Could you check a few things on this model? Use its own coordinates, in mm. A direction names the side the tool comes from. Coordinates: 2 decimals unless noted, no trailing zeros. Order: outer loops, then holes, each group sorted by start corner. A loop starts at its lowest first (then second) coordinate and runs counter-clockwise, first axis right, second up. Notation, with made-up numbers: M 52.25,-22 L 104.25,-22 A22 cw 104.25,9 Z; hole C -22,38 d4. An arc over 180 degrees is marked long. Write item = value, one per line. Start each with the question number.
from build123d import *

# Parameters (mm, degrees)
BOSS_EXTRUDE1_DEPTH = 29.5
SKETCH2_W           = 2
SKETCH2_H           = 1.8
BOSS_EXTRUDE2_DEPTH = 29.5


with BuildPart() as part:
    # Sketch1 → Boss-Extrude1 (new body)
    with BuildSketch(Plane.XY):
        Polygon((-7.65, 2.6), (2.05, 2.6), (2.05, -7), (-1.15, -7), (-1.15, -5), (0.05, -5), (0.05, 0.2), (-5.65, 0.2), (-5.65, -5), (-4.45, -5), (-4.45, -7), (-7.65, -7), align=None)
    extrude(amount=BOSS_EXTRUDE1_DEPTH)

    # Sketch2 → Boss-Extrude2 (add)
    with BuildSketch(Plane.XY.offset(29.5)):
        with Locations((1.05, 3.5)):
            Rectangle(SKETCH2_W, SKETCH2_H)
    extrude(amount=-BOSS_EXTRUDE2_DEPTH)


solid = part.part
(1) Thinking about a two-plate mould opening in Y: for faces 5 (the flat face through (-4, 2.6, 15)), 6 (the flat face through (2.05, -1, 15)), 7 (the flat face through (-0.6, -5, 14.5)), which applies, released by +Y, released by -Y, zero draft, split by the parting line, or undercut?
(2) Imagine slicing it at C-C on z = 10. List the corners of the cut face in (x, y) for me.
(3) For faces 1 (the flat face through (0.05, 3, 15)), 2 (the flat face through (-5.65, -2, 15)), 3 (the flat face through (-1.15, -6, 15)), 4 (the flat face through (-3, 1, 0)), which set-ups out of +Z, -Z, +X, -X, +Y, -Y let a thin tool reach every point of the face, with its end or its side?
(4) Imagine slicing it at D-D on x = -6.75. List the corners of the cut face in (y, z) for me, plus the area to 3 significant figures.
(5) Imagine slicing it at A-A on y = -5.75. List the corners of the cut face in (x, z) for me.
(6) Please list where these lines run through material, in increasing order: probe 1 along X at (y, z) = (0, 19); probe 2 along Y at (x, z) = (0, 12.75); probe 3 along X at (y, z) = (2.75, 20.25). Write a range as from..to.
(7) Will these pins go through, and if not, where does the flat tip stop? P1, Ø4, axis at x = -2.5, z = 14.5, coming from the +Y side; P2, Ø4.5, axis at x = -1.5, z = 18.5, coming from the -Y side; P3, Ø0.9, axis at y = 3.5, z = 15, coming from the -X side.
(8) Imagine slicing it at B-B on x = -0.5. List the corners of the cut face in (y, z) for me, plus the area to 3 significant figures.
Response:
q1.face_5 = released by +Y
q1.face_6 = zero draft
q1.face_7 = undercut
q2.outline = M -7.65,-7 L -4.45,-7 L -4.45,-5 L -5.65,-5 L -5.65,0.2 L 0.05,0.2 L 0.05,-5 L -1.15,-5 L -1.15,-7 L 2.05,-7 L 2.05,4.4 L 0.05,4.4 L 0.05,2.6 L -7.65,2.6 Z
q3.face_1 = +Z, -Z, -X, +Y
q3.face_2 = +Z, -Z
q3.face_3 = +Z, -Z, -Y
q3.face_4 = -Z, +X, -X, +Y, -Y
q4.outline = M -7,0 L 2.6,0 L 2.6,29.5 L -7,29.5 Z
q4.area = 283 mm2
q5.outline = M -7.65,0 L -4.45,0 L -4.45,29.5 L -7.65,29.5 Z; M -1.15,0 L 2.05,0 L 2.05,29.5 L -1.15,29.5 Z
q6.probe_1 = -7.65..-5.65, 0.05..2.05
q6.probe_2 = -7..-5, 0.2..2.6
q6.probe_3 = 0.05..2.05
q7.P1 = 2.6
q7.P2 = -7
q7.P3 = 0.05
q8.outline = M -7,0 L -5,0 L -5,29.5 L -7,29.5 Z; M 0.2,0 L 2.6,0 L 2.6,29.5 L 0.2,29.5 Z
q8.area = 130 mm2
